```python
from build123d import *

# Parameters (mm, degrees)
CROQUIS1_R              = 1.59
CROQUIS1_R_2            = 1.597396507
CROQUIS1_R_3            = 4
SALIENTE_EXTRUIR1_DEPTH = 5


with BuildPart() as part:
    # Croquis1 → Saliente-Extruir1 (new body)
    with BuildSketch(Plane.XY):
        with BuildLine():
            ThreePointArc((0.575431621, 26.806598054), (0.289790201, 26.858453505), (0, 26.875821538))
            ThreePointArc((0, 26.875821538), (-0.289790201, 26.858453505), (-0.575431621, 26.806598054))
            ThreePointArc((-0.575431621, 26.806598054), (-0.726756088, 26.756581913), (-0.868212659, 26.683160203))
            Line((-0.868212659, 26.683160203), (-3.655582472, 24.941297878))
            ThreePointArc((-3.655582472, 24.941297878), (-3.850805823, 24.781837219), (-3.999952041, 24.578624857))
            Line((-3.999952041, 24.578624857), (-6.759600821, 14.534111339))
            ThreePointArc((-6.759600821, 14.534111339), (-8.069386565, 11.655007451), (-10.212860864, 9.329003191))
            Line((-10.212860864, 9.329003191), (-10.213051715, 9.328852796))
            ThreePointArc((-10.213051715, 9.328852796), (-11.736097249, 6.280434064), (-10.356800654, 3.164336284))
            ThreePointArc((-10.356800654, 3.164336284), (-8.911806366, 0), (-10.356800654, -3.164336284))
            ThreePointArc((-10.356800654, -3.164336284), (-11.730778796, -6.413465762), (-9.998574535, -9.48659555))
            add(Edge.make_bspline(
                [(-4.75, -19.102398031), (-4.354825004, -14.738479929), (-6.980177997, -11.541798515), (-9.998574535, -9.48659555)],
                knots=[0, 0, 0, 0, 1, 1, 1, 1], degree=3))
            Line((-4.75, -19.102398031), (-4.75, -20))
            Line((-4.75, -20), (-5.626230736, -80))
            Line((-5.626230736, -80), (-5.626230736, -82.958659211))
            add(Edge.make_bspline(
                [(-5.626230736, -82.958659211), (-3.957996586, -86.469029482), (-1.413273472, -88.8202413), (1.317079372, -91.291125809)],
                knots=[0, 0, 0, 0, 0.775055833, 0.775055833, 0.775055833, 0.775055833], degree=3))
            Line((1.317079372, -91.291125809), (7.31863448, -96.699816586))
            Line((7.31863448, -96.699816586), (11.655892242, -91.88713778))
            Line((11.655892242, -91.88713778), (11.488752063, -91.736508564))
            Line((11.488752063, -91.736508564), (9.346047089, -89.776810767))
            ThreePointArc((9.346047089, -89.776810767), (6.105829013, -85.413576573), (5.626230736, -80))
            Line((5.626230736, -80), (4.75, -20))
            Line((4.75, -20), (4.75, -19.102398031))
            add(Edge.make_bspline(
                [(4.75, -19.102398031), (4.354825004, -14.738479929), (6.980177997, -11.541798515), (9.998574535, -9.48659555)],
                knots=[0, 0, 0, 0, 1, 1, 1, 1], degree=3))
            ThreePointArc((9.998574535, -9.48659555), (11.730778796, -6.413465762), (10.356800654, -3.164336284))
            ThreePointArc((10.356800654, -3.164336284), (8.911806366, 0), (10.356800654, 3.164336284))
            ThreePointArc((10.356800654, 3.164336284), (11.736094415, 6.280555524), (10.212860864, 9.329003191))
            ThreePointArc((10.212860864, 9.329003191), (8.069386565, 11.655007451), (6.759600821, 14.534111339))
            Line((6.759600821, 14.534111339), (3.999952041, 24.578624857))
            ThreePointArc((3.999952041, 24.578624857), (3.850805823, 24.781837219), (3.655582472, 24.941297878))
            Line((3.655582472, 24.941297878), (0.868212659, 26.683160203))
            ThreePointArc((0.868212659, 26.683160203), (0.726756088, 26.756581913), (0.575431621, 26.806598054))
        make_face()
        with Locations((-1.433916555, -83.744346036)):
            Circle(CROQUIS1_R, mode=Mode.SUBTRACT)
        with Locations((0.324013646, -73.204752137)):
            Circle(CROQUIS1_R_2, mode=Mode.SUBTRACT)
        with BuildLine():
            ThreePointArc((-5.091168825, -7.283199846), (-7.283199846, -7.283199846), (-7.283199846, -5.091168825))
            Line((-7.283199846, -5.091168825), (-6.222539674, -4.030508653))
            ThreePointArc((-6.222539674, -4.030508653), (-4.030508653, -4.030508653), (-4.030508653, -6.222539674))
            Line((-4.030508653, -6.222539674), (-5.091168825, -7.283199846))
        make_face(mode=Mode.SUBTRACT)
        with BuildLine():
            ThreePointArc((-7.283199846, 5.091168825), (-7.283199846, 7.283199846), (-5.091168825, 7.283199846))
            Line((-5.091168825, 7.283199846), (-4.030508653, 6.222539674))
            ThreePointArc((-4.030508653, 6.222539674), (-4.030508653, 4.030508653), (-6.222539674, 4.030508653))
            Line((-6.222539674, 4.030508653), (-7.283199846, 5.091168825))
        make_face(mode=Mode.SUBTRACT)
        with BuildLine():
            ThreePointArc((7.283199846, -5.091168825), (7.283199846, -7.283199846), (5.091168825, -7.283199846))
            Line((5.091168825, -7.283199846), (4.030508653, -6.222539674))
            ThreePointArc((4.030508653, -6.222539674), (4.030508653, -4.030508653), (6.222539674, -4.030508653))
            Line((6.222539674, -4.030508653), (7.283199846, -5.091168825))
        make_face(mode=Mode.SUBTRACT)
        Circle(CROQUIS1_R_3, mode=Mode.SUBTRACT)
        with BuildLine():
            Line((4.560838717, 6.752869739), (5.091168825, 7.283199846))
            ThreePointArc((5.091168825, 7.283199846), (7.283199846, 7.283199846), (7.283199846, 5.091168825))
            Line((7.283199846, 5.091168825), (6.574607513, 4.382576491))
            ThreePointArc((6.574607513, 4.382576491), (6.567912728, 4.390303583), (6.561246717, 4.398055511))
            ThreePointArc((6.561246717, 4.398055511), (4.475555235, 4.653344091), (4.560838717, 6.752869739))
        make_face(mode=Mode.SUBTRACT)
        with BuildLine():
            ThreePointArc((2.197784017, 13.915961953), (0, 11.718177935), (-2.197784017, 13.915961953))
            Line((-2.197784017, 13.915961953), (-1.25, 20.851501258))
            ThreePointArc((-1.25, 20.851501258), (-0.883883476, 21.735384735), (0, 22.101501258))
            ThreePointArc((0, 22.101501258), (0.883883476, 21.735384735), (1.25, 20.851501258))
            Line((1.25, 20.851501258), (2.197784017, 13.915961953))
        make_face(mode=Mode.SUBTRACT)
    extrude(amount=SALIENTE_EXTRUIR1_DEPTH)


solid = part.part
```
Geometry check sheet. Reference: the model listing, model coordinates, mm. A direction names the side the tool comes from. Give positions to 0.01 mm unless a question says otherwise; leave off trailing zeros. Loops run counter-clockwise (first coordinate to the right, second up) from the corner with the lowest first, then second, coordinate; pieces in that order, holes last. Notation, with made-up numbers: (14.5, 83.5) - (45.5, 83.5) arc R17 ccw to (45.5, 93.5) - close; hole circle Ø6 at (86.25, 84). An arc over 180 degrees is marked (long way). Use CSV: the item, a comma, the result in double quotes. Start each with the question number.
Q1. Section check A-A, the plane y = 0. Record the cut outline in (x, z), and give its area (3 significant figures).
Q2. Release check for a two-part mould opening along X. For faces 1 (the face through (-8.045, 11.692, 2.465)), 2 (the face through (0, -34, 5)), 3 (the face through (-0.022, -74.764, 2.465)) record: +X half, -X half, draft (parallel to the pull), parting line (faces both ways), or undercut.
Q3. Section check C-C, the plane y = -77.5. Record the cut outline in (x, z), and give its area (3 significant figures).
Q4. Scan lines: probe 1 along Y at (x, z) = (-7.25, 2.65); probe 2 along Y at (x, z) = (10.75, 0.8); probe 3 along X at (y, z) = (-6, 1.1). Record each from-to range of solid material in increasing order. Write a range as from..to.
Q5. Access from +Z, -Z, +X, -X, +Y, -Y to the whole of each face (thin tool, end or side, straight path). Record for faces 4 (the face through (-11.735, 6.33, 2.465)), 5 (the face through (0.05, 11.72, 2.46)).
Q6. Go/stop test with flat-tipped pins: pin 1 Ø2 at (y, z) = (-61, 4) entering from -X; pin 2 Ø0.7 at (y, z) = (-19.5, 2.5) entering from -X; pin 3 Ø1 at (y, z) = (-29.5, 1.5) entering from +X. Record where each tip stops, or that it passes through.
Q7. Section check B-B, the plane z = 3.65. Count the separate pieces of the cut face and the enclosed holes in it, and give its area (3 significant figures).
Findings below:
1,outline,"(-8.91, 0) - (-4, 0) - (-4, 5) - (-8.91, 5) - close; (4, 0) - (8.91, 0) - (8.91, 5) - (4, 5) - close"
1,area,"49.1 mm^2"
2,face 1,"-X half"
2,face 2,"draft"
2,face 3,"undercut"
3,outline,"(-5.59, 0) - (5.59, 0) - (5.59, 5) - (-5.59, 5) - close"
3,area,"55.9 mm^2"
4,probe 1,"y = -11.88..-7.32, -5.06..5.06, 7.32..13.15"
4,probe 2,"y = -92.89..-91.06, -8.82..-3.56, 3.56..8.82"
4,probe 3,"x = -11.73..-7.73, -3.85..3.85, 7.73..11.73"
5,face 4,"+Z, -Z, -X"
5,face 5,"+Z, -Z"
6,pin 1,"stops at x = -5.36"
6,pin 2,"stops at x = -4.75"
6,pin 3,"stops at x = 4.9"
7,separate pieces,"1"
7,enclosed holes,"8"
7,area,"1,350 mm^2"
